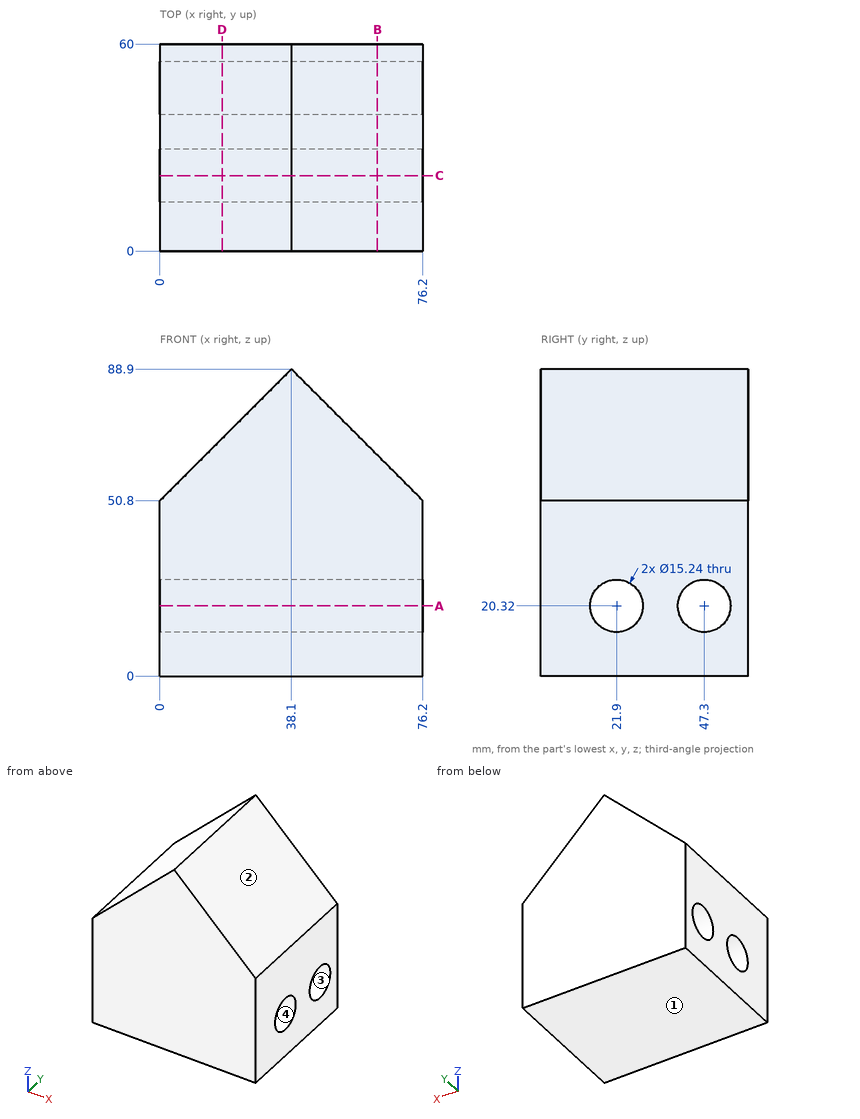
Part print with two shaded views. Sizes in mm from the minimum x, y, z corner. Give positions to 0.01 mm unless a question says otherwise; leave off trailing zeros. Order: outer loops, then holes, each group sorted by start corner. A loop starts at its lowest first (then second) coordinate and runs counter-clockwise, first axis right, second up.
(1) Saw through at D-D, the plane x = 18. Give the cut face in (y, z).
(2) Drill centre lines: L1, parallel to Y at x = 50.5, z = 26; L2, parallel to Y at x = 60, z = 23.5; L3, parallel to Z at x = 32, y = 21. Where is each one in solid material? Low to high.
(3) Mould opens along Z. For the marked faces 1, 2, 3 and 4 say: released by +Z, released by -Z, zero draft, split by the parting line, or undercut.
(4) Flat gauge pins, fed straight in: pin 1 (6 mm diameter, centred on y = 32.5, z = 77, fed in from -X); pin 2 (1.5 mm diameter, centred on x = 16, y = 32.5, fed in from -Z); pin 3 (12 mm diameter, centred on y = 26.5, z = 78.5, fed in from +X); pin 4 (8 mm diameter, centred on y = 31.5, z = 62.5, fed in from +X). Where does each tip first touch, or does it go through?
(5) Saw through at A-A, the plane z = 20.32. Give the cut face in (x, y).
(6) Saw through at B-B, the plane x = 63. Give the cut face in (y, z), then the cut area to 3 significant figures.
(7) Saw through at C-C, the plane y = 21.9. Give the cut face in (x, z).
Results found:
1. outline: (0, 0) - (60, 0) - (60, 68.8) - (0, 68.8) - close; hole circle Ø15.24 at (21.9, 20.32); hole circle Ø15.24 at (47.3, 20.32)
2. L1: y = 0 to 16.82, 26.98 to 42.22, 52.38 to 60
2. L2: y = 0 to 14.98, 28.82 to 40.38, 54.22 to 60
2. L3: z = 0 to 12.75, 27.89 to 82.8
3. face 1: released by -Z
3. face 2: released by +Z
3. face 3: undercut
3. face 4: undercut
4. pin 1: stops at x = 23.2
4. pin 2: stops at z = 0
4. pin 3: stops at x = 54.5
4. pin 4: stops at x = 68.5
5. outline: (0, 0) - (76.2, 0) - (76.2, 14.28) - (0, 14.28) - close; (0, 29.52) - (76.2, 29.52) - (76.2, 39.68) - (0, 39.68) - close; (0, 54.92) - (76.2, 54.92) - (76.2, 60) - (0, 60) - close
6. outline: (0, 0) - (60, 0) - (60, 64) - (0, 64) - close; hole circle Ø15.24 at (21.9, 20.32); hole circle Ø15.24 at (47.3, 20.32)
6. area: 3,480 mm2
7. outline: (0, 0) - (76.2, 0) - (76.2, 12.7) - (0, 12.7) - close; (0, 27.94) - (76.2, 27.94) - (76.2, 50.8) - (38.1, 88.9) - (0, 50.8) - close
